Part model, mm, in its own coordinate system. A direction names the side the tool comes from. Coordinates: 2 decimals unless noted, no trailing zeros. Write each loop counter-clockwise with the first axis right and the second up, starting at its lowest first coordinate (ties: lowest second). Pieces come first, ordered by that corner, then holes. Notation, with made-up numbers: (-28.75, 35) -> (6.25, 35) arc R28 cw to (6.25, 67) -> close; hole circle Ø7 at (-15, 24). An arc over 180 degrees is marked (long way). Write item = value, one per line. Start each with the question number.
Q1. Probe line 1 (Z direction, x = -240.5, y = -330.5); line 2 (Y direction, x = -451.5, z = -435); line 3 (X direction, y = -352.5, z = -528). List the from-to ranges inside material, lowest first.
Q2. Band-saw the part on B-B, the plane z = -436. List the corners of the cut face in (x, y), plus the area to 3 significant figures.
Q3. Tool access for faces 4 (the flat face through (-283, 0, -325)), 5 (the flat face through (-127, -501, -319.311)), 6 (the flat face through (-290, -12.7, -325)): list every direction of +Z, -Z, +X, -X, +Y, -Y with a clear straight run to the whole face (end or side of a thin tool).
Q4. Band-saw the part on A-A, the plane x = -474. List the corners of the cut face in (y, z).
Q5. Pin check, flat tips, straight feed: P1, Ø3, axis at y = -178.5, z = -469, coming from the +X side; P2, Ø14, axis at x = -6, z = -358.5, coming from the -Y side; P3, Ø1.5, axis at y = -211, z = -448.5, coming from the -X side; P4, Ø10, axis at y = -500, z = -389, coming from the +X side. Stop position of each tip, or through.
Q6. Band-saw the part on D-D, the plane y = -57.5. List the corners of the cut face in (x, z), plus the area to 3 significant figures.
Q7. Pull direction Z, two halves, no side cores. Call faces 1 (the flat face through (0, -250, -332)), 2 (the flat face through (-290, -251, -569.905)), 3 (the flat face through (-283, -250, -582.605)): released by +Z, released by -Z, zero draft, split by the parting line, or undercut.
Q8. Band-saw the part on C-C, the plane z = -155. List the corners of the cut face in (x, y), plus the area to 3 significant figures.
from build123d import *

# Parameters (mm, degrees)
F0_W     = 558.8
F0_H     = 508
F1_DEPTH = 508
F2_T     = -12.7
F5_W     = 250.6727086544
F5_H     = 137.283227253
F6_DEPTH = 25.4


# Not quite as in the source:
# - the program builds the solid bodies; features that only make, move or delete a surface that nothing else refers to are left out


with BuildPart() as f1:
    # F0 (on Front) → F1 (new body)
    with BuildSketch(Plane.XZ):
        with Locations((-279.4, -328.6047284609)):
            Rectangle(F0_W, F0_H)
    extrude(amount=F1_DEPTH)

    # F2
    f2_openings = [f1.faces().sort_by_distance(p)[0] for p in [
        (-558.8, -254, -328.604728),
    ]]
    offset(amount=F2_T, openings=f2_openings)

    # F5 (on face) → F6 (cut)
    with BuildSketch(Plane.XZ.offset(508)):
        with Locations((-125.3363543272, -387.9528045654)):
            Rectangle(F5_W, F5_H)
    extrude(amount=-F6_DEPTH, mode=Mode.SUBTRACT)


solid = f1.part
Ans:
q1.line_1 = -582.6 to -569.9, -87.3 to -74.6
q1.line_2 = -508 to -495.3, -12.7 to 0
q1.line_3 = -12.7 to 0
q2.outline = (-558.8, -508) -> (-250.67, -508) -> (-250.67, -495.3) -> (-558.8, -495.3) -> close; (-558.8, -12.7) -> (-12.7, -12.7) -> (-12.7, -482.6) -> (0, -482.6) -> (0, 0) -> (-558.8, 0) -> close
q2.area = 17,000 mm2
q3.face_4 = +Z, -Z, +X, -X, +Y
q3.face_5 = +X, -Y
q3.face_6 = -X
q4.outline = (-508, -582.6) -> (0, -582.6) -> (0, -74.6) -> (-508, -74.6) -> close; hole (-495.3, -569.9) -> (-12.7, -569.9) -> (-12.7, -87.3) -> (-495.3, -87.3) -> close
q5.P1 = 0
q5.P2 = -482.6
q5.P3 = -12.7
q5.P4 = -250.67
q6.outline = (-558.8, -582.6) -> (0, -582.6) -> (0, -74.6) -> (-558.8, -74.6) -> (-558.8, -87.3) -> (-12.7, -87.3) -> (-12.7, -569.9) -> (-558.8, -569.9) -> close
q6.area = 20,300 mm2
q7.face_1 = zero draft
q7.face_2 = undercut
q7.face_3 = released by -Z
q8.outline = (-558.8, -508) -> (0, -508) -> (0, 0) -> (-558.8, 0) -> (-558.8, -12.7) -> (-12.7, -12.7) -> (-12.7, -495.3) -> (-558.8, -495.3) -> close
q8.area = 20,300 mm2
